Source: CAD feature listing. Evaluate the final solid. Frame: model axes, mm. Face numbers are marked on the shaded views. A direction names the side the tool comes from. Give positions to 0.01 mm unless a question says otherwise; leave off trailing zeros. Loops run counter-clockwise (first coordinate to the right, second up) from the corner with the lowest first, then second, coordinate; pieces in that order, holes last. Notation, with made-up numbers: M -33,15 L 12,15 A25 cw 12,32 Z; hole C -6,54.25 d1. An arc over 180 degrees is marked long. Write item = value, one per line.
from build123d import *

# Parameters (mm, degrees)
FILLET_1_R          = 0.475
CUT_EXTRUDE_1_DEPTH = 1


with BuildPart() as part:
    # 草图1 → 旋转1 (revolve)
    with BuildSketch(Plane(origin=(0, 0, 0), x_dir=(0, 0, -1), z_dir=(1, 0, 0))):
        Polygon((0, 0), (0, 2.95), (0.95, 2.95), (0.95, 1.5), (10.95, 1.5), (10.95, 0), align=None)
    revolve(axis=Axis((0, 0, -10.95), (0, 0, 1)))

    # 圆角1
    fillet_1_edges = [part.edges().sort_by_distance(p)[0] for p in [
        (0, -2.95, -0.95),
        (0, -2.95, 0),
    ]]
    fillet(fillet_1_edges, radius=FILLET_1_R - 0.0001)  # a hair under: the kernel refuses the full size

    # 草图2 → 切除-拉伸1 (cut)
    with BuildSketch(Plane.XY):
        Polygon((0.577350269, 1), (-0.577350269, 1), (-1.154700538, 0), (-0.577350269, -1), (0.577350269, -1), (1.154700538, 0), align=None)
    extrude(amount=-CUT_EXTRUDE_1_DEPTH, mode=Mode.SUBTRACT)


solid = part.part
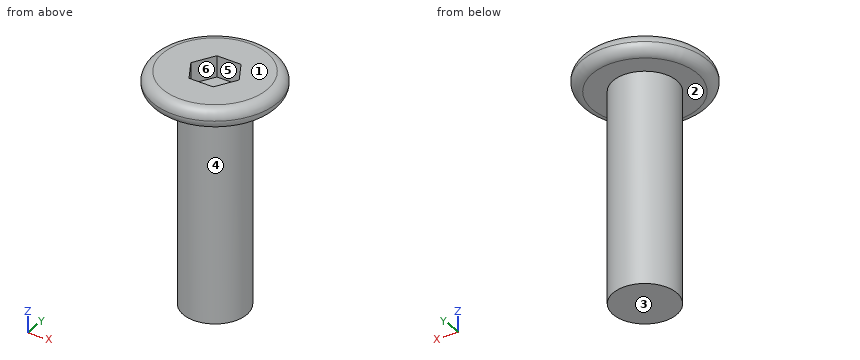
1. First-contact query: pin 1 Ø1 at (y, z) = (1.5, -3.5) entering from -X; pin 2 Ø3 at (x, y) = (1.5, 0.5) entering from +Z; pin 3 Ø3 at (x, z) = (0.5, -9.5) entering from +Y; pin 4 Ø3 at (y, z) = (-1.5, -4.5) entering from +X. Flat tips, straight axial feed; report the tip coordinate or a pass-through.
Derived:
pin_1 = -1.12
pin_2 = 0
pin_3 = 1.5
pin_4 = 1.5
2. Material intervals for probe 1 along X at (y, z) = (0, -3); probe 2 along Z at (x, y) = (0.95, -2); probe 3 along Z at (x, y) = (0.9, 0.35), sorted ascending. Write a range as from..to.
Derived:
probe_1 = -1.5..1.5
probe_2 = -0.95..0
probe_3 = -10.95..-1
3. Reachability of the marked faces 1 and 2 from +Z, -Z, +X, -X, +Y, -Y: full face, straight path, thin tool, end or side. Return the list, or none.
Derived:
face_1 = +Z, +X, -X, +Y, -Y
face_2 = -Z
4. Cut plane B-B, the plane z = -10. Return the cut outline in (x, y), then the cut area to 3 significant figures.
Derived:
outline = C 0,0 d3
area = 7.07 mm²
5. Pull-direction query (Y, two-part tool) for the marked faces 3, 4, 5 and 6; classes: +Y half, -Y half, draft (parallel to the pull), parting line (faces both ways), or undercut.
Derived:
face_3 = draft
face_4 = parting line
face_5 = undercut
face_6 = undercut
